```python
from build123d import *

# Parameters (mm, degrees)
BOSS_EXTRUDE1_DEPTH     = 20
SKETCH10_R              = 2.5
CUT_EXTRUDE1_DEPTH      = 90
CUT_EXTRUDE1_DEPTH_BACK = 479
SKETCH11_R              = 2.5
CUT_EXTRUDE2_DEPTH      = 47
CUT_EXTRUDE2_DEPTH_BACK = 47


with BuildPart() as part:
    # Sketch9 → Boss-Extrude1 (new body)
    with BuildSketch(Plane.XY):
        Polygon((-158.103055268, -153.493142729), (-158.103055268, -113.493142729), (-26.676129575, 65.42293593), (53.323870425, 65.42293593), (184.750796118, -113.493142729), (184.750796118, -153.493142729), (186.750796118, -153.493142729), (186.750796118, -112.83750963), (54.33633476, 67.42293593), (-27.68859391, 67.42293593), (-160.103055268, -112.83750963), (-160.103055268, -153.493142729), align=None)
    extrude(amount=BOSS_EXTRUDE1_DEPTH)

    # Sketch10 → Cut-Extrude1 (cut, two sides)
    with BuildSketch(Plane(origin=(186.750796118, 0, 0), x_dir=(0, 0, -1), z_dir=(1, 0, 0))) as cut_extrude1_sk:
        with Locations((-9.534610309, -143.493142729)):
            Circle(SKETCH10_R)
    extrude(amount=CUT_EXTRUDE1_DEPTH, mode=Mode.SUBTRACT)
    extrude(cut_extrude1_sk.sketch, amount=-CUT_EXTRUDE1_DEPTH_BACK, mode=Mode.SUBTRACT)

    # Sketch11 → Cut-Extrude2 (cut, two sides)
    with BuildSketch(Plane(origin=(0, 67.42293593, 0), x_dir=(1, 0, 0), z_dir=(0, 1, 0))) as cut_extrude2_sk:
        with Locations((-7.68859391, -10)):
            Circle(SKETCH11_R)
        with Locations((34.33633476, -10)):
            Circle(SKETCH11_R)
        with Locations((13.31140609, -9.999992232)):
            Circle(SKETCH11_R)
    extrude(amount=CUT_EXTRUDE2_DEPTH, mode=Mode.SUBTRACT)
    extrude(cut_extrude2_sk.sketch, amount=-CUT_EXTRUDE2_DEPTH_BACK, mode=Mode.SUBTRACT)


solid = part.part
```
Build history of the part. All positions in model axes, mm. A direction names the side the tool comes from. Round coordinates to 2 decimals unless told otherwise and drop trailing zeros. Loops run counter-clockwise (first coordinate to the right, second up) from the corner with the lowest first, then second, coordinate; pieces in that order, holes last.
Item 1: Two-plate mould, pull along X, no slides. Class faces 3 (the face through (121.47, -23.97, 9.86)), 4 (the face through (14, 67.423, 5)), 5 (the face through (-93.31, -25.29, 9.86)): released by +X, released by -X, zero draft, split by the parting line, or undercut.
Item 2: Drill centre lines: line 1 along X through (y, z) = (66.5, 10); line 2 along X through (y, z) = (66.85, 10); line 3 along X through (y, z) = (-135.5, 6). Where is each one in solid material? Low to high.
Item 3: Saw through at D-D (x = 47.5). List the corners of the cut face in (y, z).
Item 4: Saw through at C-C (x = 106). List the corners of the cut face in (y, z), then the cut area to 3 significant figures.
Item 5: Saw through at A-A (z = 4). List the corners of the cut face in (x, y), then the cut area to 3 significant figures.
Item 6: Pin check, flat tips, straight feed: P1, Ø12, axis at x = 114, y = 1.5, coming from the +Z side (3 decimals); P2, Ø4, axis at y = -13, z = 10, coming from the -X side; P3, Ø1.5, axis at x = -28.5, z = 9.5, coming from the -Y side; P4, Ø6, axis at y = -19.5, z = 13.5, coming from the +X side. Stop position of each tip, or through.
Item 7: Saw through at B-B (y = -27). List the corners of the cut face in (x, z), then the cut area to 3 significant figures.
Item 8: Which spindle directions (+Z, -Z, +X, -X, +Y, -Y) get a long thin tool onto all of the face, cutting with end or side? Do faces 1 (the face through (13, 65.423, 5)), 2 (the face through (186.751, -133, 10)). Say none if no direction does.
Worked answers:
1. face 3: released by +X
1. face 4: zero draft
1. face 5: undercut
2. line 1: x = -28.37 to -10.19, -5.19 to 10.81, 15.81 to 31.84, 36.84 to 55.01
2. line 2: x = -28.11 to -10.19, -5.19 to 10.81, 15.81 to 31.84, 36.84 to 54.76
2. line 3: x = -160.1 to -158.1, 184.75 to 186.75
3. outline: (65.42, 0) - (67.42, 0) - (67.42, 20) - (65.42, 20) - close
4. outline: (-6.29, 0) - (-2.91, 0) - (-2.91, 20) - (-6.29, 20) - close
4. area: 67.6 mm2
5. outline: (-160.1, -153.49) - (-158.1, -153.49) - (-158.1, -113.49) - (-26.68, 65.42) - (53.32, 65.42) - (184.75, -113.49) - (184.75, -153.49) - (186.75, -153.49) - (186.75, -112.84) - (54.34, 67.42) - (-27.69, 67.42) - (-160.1, -112.84) - close
5. area: 1,210 mm2
6. P1: passes through
6. P2: stops at x = -88.23
6. P3: stops at y = 61.92
6. P4: stops at x = 120.39
7. outline: (-97.05, 0) - (-94.57, 0) - (-94.57, 20) - (-97.05, 20) - close; (121.22, 0) - (123.7, 0) - (123.7, 20) - (121.22, 20) - close
7. area: 99.3 mm2
8. face 1: +Z, -Z, -Y
8. face 2: +Z, -Z, +X, +Y, -Y
